Part model, mm, in its own coordinate system. A direction names the side the tool comes from. Coordinates: 2 decimals unless noted, no trailing zeros. Write each loop counter-clockwise with the first axis right and the second up, starting at its lowest first coordinate (ties: lowest second). Pieces come first, ordered by that corner, then holes. Notation, with made-up numbers: (56.5, -30) -> (91.5, -30) arc R26 cw to (91.5, 9) -> close; hole circle Ø8 at (71, 81.5). An arc over 180 degrees is marked (long way). Write item = value, one per line.
from build123d import *

# Parameters (mm, degrees)
SKETCH_1_W          = 540
SKETCH_1_H          = 265
SKETCH_1_R          = 13
EXTRUDE_551_DEPTH   = 11.5
SKETCH_2_W          = 540
SKETCH_2_H          = 11.5
EXTRUDE_1_DEPTH     = 77.5
CUT_EXTRUDE_1_DEPTH = 609.067430471
SKETCH_4_R          = 13
CUT_EXTRUDE_2_DEPTH = 609.067430471
SKETCH_5_W          = 14
SKETCH_5_H          = 253.5
EXTRUDE_2_DEPTH     = 208.5
SKETCH_6_R          = 13
CUT_EXTRUDE_3_DEPTH = 442.988687638


with BuildPart() as part:
    # 草图1 → Extrude 551 (new body)
    with BuildSketch(Plane.XY):
        with Locations((270, 132.5)):
            Rectangle(SKETCH_1_W, SKETCH_1_H)
        with Locations((97.46594539, 108.46594539)):
            Circle(SKETCH_1_R, mode=Mode.SUBTRACT)
        with Locations((40.897402896, 51.897402896)):
            Circle(SKETCH_1_R, mode=Mode.SUBTRACT)
        with Locations(Location((499.102597104, 51.897402896, 0), (0, 0, 180))):
            Circle(SKETCH_1_R, mode=Mode.SUBTRACT)
        with Locations(Location((402.170987639, 92.261534081, 0), (0, 0, 180))):
            Circle(SKETCH_1_R, mode=Mode.SUBTRACT)
        with Locations((230, 121)):
            Circle(SKETCH_1_R, mode=Mode.SUBTRACT)
        with Locations((230, 41)):
            Circle(SKETCH_1_R, mode=Mode.SUBTRACT)
        with Locations(Location((310, 41, 0), (0, 0, 180))):
            Circle(SKETCH_1_R, mode=Mode.SUBTRACT)
        with Locations(Location((310, 121, 0), (0, 0, 180))):
            Circle(SKETCH_1_R, mode=Mode.SUBTRACT)
        with Locations((137.829012361, 92.261534081)):
            Circle(SKETCH_1_R, mode=Mode.SUBTRACT)
        with Locations(Location((442.53405461, 108.46594539, 0), (0, 0, 180))):
            Circle(SKETCH_1_R, mode=Mode.SUBTRACT)
    extrude(amount=EXTRUDE_551_DEPTH)

    # 草图2 → 凸台-拉伸1 (add)
    with BuildSketch(Plane.XY.offset(11.5)):
        with Locations((270, 259.25)):
            Rectangle(SKETCH_2_W, SKETCH_2_H)
    extrude(amount=EXTRUDE_1_DEPTH)

    # 草图3 → 切除-拉伸1 (cut, through all)
    with BuildSketch(Plane(origin=(0, 265, 0), x_dir=(-1, 0, 0), z_dir=(0, 1, 0))):
        Polygon((0, 0), (-100, 89), (0, 89), align=None)
        Polygon((-540, 0), (-440, 89), (-540, 89), align=None)
    extrude(amount=-CUT_EXTRUDE_1_DEPTH, mode=Mode.SUBTRACT)

    # 草图4 → 切除-拉伸2 (cut, through all)
    with BuildSketch(Plane(origin=(0, 265, 0), x_dir=(-1, 0, 0), z_dir=(0, 1, 0))):
        with Locations(Location((-210, 50, 0), (0, 0, 90))):
            Circle(SKETCH_4_R)
        with Locations(Location((-130, 50, 0), (0, 0, 90))):
            Circle(SKETCH_4_R)
        with Locations(Location((-410, 50, 0), (0, 0, 90))):
            Circle(SKETCH_4_R)
        with Locations(Location((-330, 50, 0), (0, 0, 90))):
            Circle(SKETCH_4_R)
    extrude(amount=-CUT_EXTRUDE_2_DEPTH, mode=Mode.SUBTRACT)

    # 草图5 → 凸台-拉伸2 (add)
    with BuildSketch(Plane.XY.offset(11.5)):
        with Locations((270, 126.75)):
            Rectangle(SKETCH_5_W, SKETCH_5_H)
    extrude(amount=EXTRUDE_2_DEPTH)

    # 草图6 → 切除-拉伸3 (cut, through all)
    with BuildSketch(Plane(origin=(277, 0, 0), x_dir=(0, 0, -1), z_dir=(1, 0, 0))):
        with Locations((-115.676148082, 138.142814541)):
            Circle(SKETCH_6_R)
        with Locations((-175.462621788, 84.986652509)):
            Circle(SKETCH_6_R)
        with Locations((-68.377294113, 126.911974174)):
            Circle(SKETCH_6_R)
        Polygon((-89, 253.5), (-220, 93.5), (-220, 253.5), align=None)
        Polygon((-220, 45), (0, 0), (-220, 0), align=None)
    extrude(amount=-CUT_EXTRUDE_3_DEPTH, mode=Mode.SUBTRACT)


solid = part.part
Q1. Saw through at B-B on z = 50. Give the cut face in (x, y), and give its area (3 significant figures).
Model answer:
outline = (56.18, 253.5) -> (117, 253.5) -> (117, 265) -> (56.18, 265) -> close; (143, 253.5) -> (197, 253.5) -> (197, 265) -> (143, 265) -> close; (223, 253.5) -> (263, 253.5) -> (263, 10.23) -> (277, 10.23) -> (277, 253.5) -> (317, 253.5) -> (317, 265) -> (223, 265) -> close; (343, 253.5) -> (397, 253.5) -> (397, 265) -> (343, 265) -> close; (423, 253.5) -> (483.82, 253.5) -> (483.82, 265) -> (423, 265) -> close
area = 7,130 mm²
Q2. Pin check, flat tips, straight feed: pin 1 (23.5 mm diameter, centred on x = 40.9, y = 51.9, fed in from +Z); pin 2 (12 mm diameter, centred on x = 193.5, y = 128, fed in from +Z); pin 3 (3 mm diameter, centred on y = 217.5, z = 62.5, fed in from +X); pin 4 (12.5 mm diameter, centred on x = 298, y = 258.5, fed in from +Z). Stop position of each tip, or through.
Model answer:
pin_1 = through
pin_2 = 11.5
pin_3 = 277
pin_4 = 89
Q3. Saw through at C-C on x = 310. Give the cut face in (y, z), and give its area (3 significant figures).
Model answer:
outline = (0, 0) -> (28, 0) -> (28, 11.5) -> (0, 11.5) -> close; (54, 0) -> (108, 0) -> (108, 11.5) -> (54, 11.5) -> close; (134, 0) -> (265, 0) -> (265, 89) -> (253.5, 89) -> (253.5, 11.5) -> (134, 11.5) -> close
area = 3,340 mm²
Q4. Probe line 1 (Y direction, x = 230, z = 4); line 2 (Z direction, x = 445.5, y = 133); line 3 (X direction, y = 78, z = 186.5). List the from-to ranges inside material, lowest first. Write a range as from..to.
Model answer:
line_1 = 0.82..28, 54..108, 134..265
line_2 = 0..11.5
line_3 = 263..277
Q5. Which spindle directions (+Z, -Z, +X, -X, +Y, -Y) get a long thin tool onto all of the face, cutting with end or side? Do faces 1 (the face through (164, 253.5, 50)), 2 (the face through (373, 253.5, 50)), 3 (the face through (12.73, 152.75, 11.33)). Say none if no direction does.
Model answer:
face_1 = +Z, -X, -Y
face_2 = +Z, +X, -Y
face_3 = +Z, -X, +Y, -Y
Q6. Mould opens along X. For faces 4 (the face through (136, 130, 11.5)), 5 (the face through (217.013, 41.572, 5.67)), 6 (the face through (527.27, 152.75, 11.33)) say: released by +X, released by -X, zero draft, split by the parting line, or undercut.
Model answer:
face_4 = zero draft
face_5 = undercut
face_6 = released by +X
Q7. Saw through at D-D on y = 183. Give the cut face in (x, z), and give its area (3 significant figures).
Model answer:
outline = (0, 0) -> (540, 0) -> (527.08, 11.5) -> (277, 11.5) -> (277, 146.72) -> (263, 146.72) -> (263, 11.5) -> (12.92, 11.5) -> close
area = 7,950 mm²
Q8. Saw through at A-A on x = 210. Give the cut face in (y, z).
Model answer:
outline = (0, 0) -> (265, 0) -> (265, 37) -> (253.5, 37) -> (253.5, 11.5) -> (2.35, 11.5) -> close; (253.5, 63) -> (265, 63) -> (265, 89) -> (253.5, 89) -> close
